from build123d import *

# Parameters (mm, degrees)
SKETCH1_W                = 27
SKETCH1_H                = 10.8
BOSS_EXTRUDE1_DEPTH      = 12
SKETCH2_W                = 3.9
SKETCH2_H                = 10.8
CUT_EXTRUDE1_DEPTH       = 4
SKETCH3_W                = 3.9
SKETCH3_H                = 10.8
CUT_EXTRUDE2_DEPTH       = 4
CUT_EXTRUDE3_DEPTH       = 31.160238726
CUT_EXTRUDE3_DEPTH_BACK  = 31.160238726
SKETCH4_R                = 1.1
CUT_EXTRUDE4_DEPTH       = 31.160238726
CUT_EXTRUDE4_DEPTH_BACK  = 31.160238726
SKETCH5_R                = 1.1
CUT_EXTRUDE5_DEPTH       = 6.5
SKETCH7_OUTSIDE_W        = 35.292
SKETCH7_OUTSIDE_H        = 19.092
SKETCH7_OUTSIDE_W_2      = 19.2
SKETCH7_OUTSIDE_H_2      = 8
CUT_EXTRUDE6_DEPTH       = 4
BOSS_EXTRUDE2_DEPTH      = 2.18
BOSS_EXTRUDE2_DEPTH_BACK = 2.18
SKETCH8_W                = 9.84
SKETCH8_H                = 3.4
SKETCH9_W                = 9.84
SKETCH9_H                = 3.4
SKETCH9_W_2              = 8.64
SKETCH9_H_2              = 2.4
CUT_EXTRUDE7_DEPTH       = 3.5


with BuildPart() as part:
    # Sketch1 → Boss-Extrude1 (new body)
    with BuildSketch(Plane(origin=(0, 0, 0), x_dir=(1, 0, 0), z_dir=(0, 1, 0))):
        with Locations((13.5, 5.4)):
            Rectangle(SKETCH1_W, SKETCH1_H)
    extrude(amount=BOSS_EXTRUDE1_DEPTH)

    # Sketch2 → Cut-Extrude1 (cut)
    with BuildSketch(Plane(origin=(0, 12, 0), x_dir=(1, 0, 0), z_dir=(0, 1, 0))):
        with Locations((1.95, 5.4)):
            Rectangle(SKETCH2_W, SKETCH2_H)
    extrude(amount=-CUT_EXTRUDE1_DEPTH, mode=Mode.SUBTRACT)

    # Sketch3 → Cut-Extrude2 (cut)
    with BuildSketch(Plane(origin=(0, 12, 0), x_dir=(1, 0, 0), z_dir=(0, 1, 0))):
        with Locations((25.05, 5.4)):
            Rectangle(SKETCH3_W, SKETCH3_H)
    extrude(amount=-CUT_EXTRUDE2_DEPTH, mode=Mode.SUBTRACT)

    # Sketch4 → Cut-Extrude3 (cut, two sides: drawn at the far end of the back side and taken through both)
    with BuildSketch(Plane(origin=(0, 8, 0), x_dir=(1, 0, 0), z_dir=(0, 1, 0)).offset(-CUT_EXTRUDE3_DEPTH_BACK)):
        with Locations(Location((25.2, 1.8, 0), (0, 0, 270))):
            Circle(SKETCH4_R)
    extrude(amount=CUT_EXTRUDE3_DEPTH + CUT_EXTRUDE3_DEPTH_BACK, mode=Mode.SUBTRACT)

    # Sketch5 → Cut-Extrude4 (cut, two sides: drawn at the far end of the back side and taken through both)
    with BuildSketch(Plane(origin=(0, 8, 0), x_dir=(1, 0, 0), z_dir=(0, 1, 0)).offset(-CUT_EXTRUDE4_DEPTH_BACK)):
        with Locations(Location((1.8, 9, 0), (0, 0, 270))):
            Circle(SKETCH5_R)
    extrude(amount=CUT_EXTRUDE4_DEPTH + CUT_EXTRUDE4_DEPTH_BACK, mode=Mode.SUBTRACT)

    # Sketch6 → Cut-Extrude5 (cut)
    with BuildSketch(Plane(origin=(0, 8, 0), x_dir=(1, 0, 0), z_dir=(0, 1, 0))):
        with BuildLine():
            Line((1.8, 6.9), (0, 6.9))
            Line((0, 6.9), (0, 10.8))
            Line((0, 10.8), (3.9, 10.8))
            Line((3.9, 10.8), (3.9, 9))
            ThreePointArc((3.9, 9), (3.28492424, 7.51507576), (1.8, 6.9))
        make_face()
        with BuildLine():
            Line((25.2, 3.9), (27, 3.9))
            Line((27, 3.9), (27, 0))
            Line((27, 0), (23.1, 0))
            Line((23.1, 0), (23.1, 1.8))
            ThreePointArc((23.1, 1.8), (23.71507576, 3.28492424), (25.2, 3.9))
        make_face()
    extrude(amount=-CUT_EXTRUDE5_DEPTH, mode=Mode.SUBTRACT)

    # Sketch7 outside → Cut-Extrude6 (cut)
    with BuildSketch(Plane(origin=(0, 12, 0), x_dir=(1, 0, 0), z_dir=(0, 1, 0))):
        with Locations((13.5, 5.4)):
            Rectangle(SKETCH7_OUTSIDE_W, SKETCH7_OUTSIDE_H)
        with Locations((13.5, 5.4)):
            Rectangle(SKETCH7_OUTSIDE_W_2, SKETCH7_OUTSIDE_H_2, mode=Mode.SUBTRACT)
    extrude(amount=-CUT_EXTRUDE6_DEPTH, mode=Mode.SUBTRACT)

    # Sketch8 → Boss-Extrude2 (add, two sides: drawn at the far end of the back side and taken through both)
    with BuildSketch(Plane.XZ.offset(-BOSS_EXTRUDE2_DEPTH_BACK)):
        with Locations((5.17, 0.7)):
            Rectangle(SKETCH8_W, SKETCH8_H)
    extrude(amount=BOSS_EXTRUDE2_DEPTH + BOSS_EXTRUDE2_DEPTH_BACK)

    # Sketch9 → Cut-Extrude7 (cut)
    with BuildSketch(Plane.XZ.offset(2.18)):
        with Locations((5.17, 0.7)):
            Rectangle(SKETCH9_W, SKETCH9_H)
        with Locations((5.17, 0.7)):
            Rectangle(SKETCH9_W_2, SKETCH9_H_2, mode=Mode.SUBTRACT)
    extrude(amount=-CUT_EXTRUDE7_DEPTH, mode=Mode.SUBTRACT)


solid = part.part
Part model, mm, in its own coordinate system. A direction names the side the tool comes from. Give positions to 0.01 mm unless a question says otherwise; leave off trailing zeros. Write each loop counter-clockwise with the first axis right and the second up, starting at its lowest first coordinate (ties: lowest second). Pieces come first, ordered by that corner, then holes.
1) Which spindle directions (+Z, -Z, +X, -X, +Y, -Y) get a long thin tool onto all of the face, cutting with end or side? Do faces 1 (the face through (10.09, 0.7, -0.5)), 2 (the face through (13, 10, -1.4)), 3 (the face through (24, 1.5, -1)), 4 (the face through (5, 1, -1)), 5 (the face through (0.25, 2, 1)). Say none if no direction does.
Resolved:
face 1: +Z, -Y
face 2: +Z, +X, -X, +Y
face 3: +Z, +X, +Y
face 4: -Y
face 5: +Z, -X, +Y, -Y
2) Pin check, flat tips, straight feed: pin 1 (2 mm diameter, centred on x = 1, y = 5.5, fed in from -Z); pin 2 (2 mm diameter, centred on x = 15, y = 10.5, fed in from +Z); pin 3 (2.5 mm diameter, centred on y = -1.5, z = 0.5, fed in from -X); pin 4 (1.2 mm diameter, centred on x = 1.5, z = -9, fed in from +Y). Stop position of each tip, or through.
Resolved:
pin 1: stops at z = -6.91
pin 2: stops at z = -1.4
pin 3: stops at x = 0.85
pin 4: passes through
3) Probe L1, parallel to Z at x = 1.8, y = 0.7; L2, parallel to Z at x = 25.2, y = 1.25; L3, parallel to X at y = 0.3, z = -9. List the from-to ranges inside material, lowest first.
Resolved:
L1: z = -10.8 to -10.1, -7.9 to -1, -0.5 to 1.9
L2: z = -10.8 to -2.9, -0.7 to 0
L3: x = 0 to 0.7, 2.9 to 27
4) Two-plate mould, pull along Z, no slides. Class faces 6 (the face through (3.3, 4.8, -7.53)), 7 (the face through (26, 5, -3.9)), 8 (the face through (19, 8, -10)), 9 (the face through (5.1, 1.32, 2.1)): released by +Z, released by -Z, zero draft, split by the parting line, or undercut.
Resolved:
face 6: released by -Z
face 7: released by +Z
face 8: zero draft
face 9: undercut
5) Cut at A-A on x = 12.75. Write the cut outline in (y, z).
Resolved:
outline: (0, -10.8) - (8, -10.8) - (8, -9.4) - (12, -9.4) - (12, -1.4) - (8, -1.4) - (8, 0) - (0, 0) - close
6) Cut at C-C on y = 5. Write the cut outline in (x, z), then the cut area to 3 significant figures.
Resolved:
outline: (0, -6.9) - (1.8, -6.9) arc R2.1 cw to (3.9, -9) - (3.9, -10.8) - (27, -10.8) - (27, -3.9) - (25.2, -3.9) arc R2.1 cw to (23.1, -1.8) - (23.1, 0) - (0, 0) - close
area: 263 mm2
7) Cut at B-B on z = 1. Write the cut outline in (x, y), then the cut area to 3 significant figures.
Resolved:
outline: (0.25, 1.32) - (0.85, 1.32) - (0.85, -2.18) - (9.49, -2.18) - (9.49, 1.32) - (10.09, 1.32) - (10.09, 2.18) - (0.25, 2.18) - close
area: 38.7 mm2
8) Cut at D-D on x = 3.5. Write the cut outline in (y, z), then the cut area to 3 significant figures.
Resolved:
outline: (-2.18, -0.5) - (1.32, -0.5) - (1.32, -1) - (0, -1) - (0, -10.8) - (1.5, -10.8) - (1.5, -7.77) - (8, -7.77) - (8, 0) - (2.18, 0) - (2.18, 2.4) - (1.32, 2.4) - (1.32, 1.9) - (-2.18, 1.9) - close
area: 75.8 mm2
